```python
from build123d import *

# Parameters (mm, degrees)
BOSS_EXTRUDE1_DEPTH = 10
CHAMFER1_SIZE       = 1


with BuildPart() as part:
    # Sketch1 → Revolve1 (revolve)
    with BuildSketch(Plane.XY, mode=Mode.PRIVATE) as revolve1_sk:
        with BuildLine():
            Line((0, 0), (0, 15))
            Line((0, 15), (14.56869778, 15))
            ThreePointArc((14.56869778, 15), (15.493526394, 14.380384062), (15.27227791, 13.289384069))
            Line((15.27227791, 13.289384069), (12.24641987, 10.29348502))
            ThreePointArc((12.24641987, 10.29348502), (12.027075266, 9.967849524), (11.95, 9.582869089))
            Line((11.95, 9.582869089), (11.95, 5.417130911))
            ThreePointArc((11.95, 5.417130911), (12.027075266, 5.032150476), (12.24641987, 4.70651498))
            Line((12.24641987, 4.70651498), (15.27227791, 1.710615931))
            ThreePointArc((15.27227791, 1.710615931), (15.493526394, 0.619615938), (14.56869778, 0))
            Line((14.56869778, 0), (0, 0))
        make_face()
    revolve(revolve1_sk.sketch.rotate(Axis((-3.05, 12, 0), (0, -1, 0)), 180), axis=Axis((-3.05, 12, 0), (0, -1, 0)))

    # Sketch2 → Boss-Extrude1 (add)
    with BuildSketch(Plane(origin=(0, 15, 0), x_dir=(1, 0, 0), z_dir=(0, 1, 0))):
        with BuildLine():
            ThreePointArc((0, 0), (-0.18033103, 1.033198916), (-0.7, 1.94422221))
            Line((-0.7, 1.94422221), (-0.7, -1.94422221))
            ThreePointArc((-0.7, -1.94422221), (-0.18033103, -1.033198916), (0, 0))
        make_face()
    extrude(amount=-BOSS_EXTRUDE1_DEPTH)

    # Chamfer1
    chamfer1_edges = [part.edges().sort_by_distance(p)[0] for p in [
        (-4.083198916, 15, -2.86966897),
        (-0.7, 15, 0),
    ]]
    chamfer(chamfer1_edges, length=CHAMFER1_SIZE)


solid = part.part
```
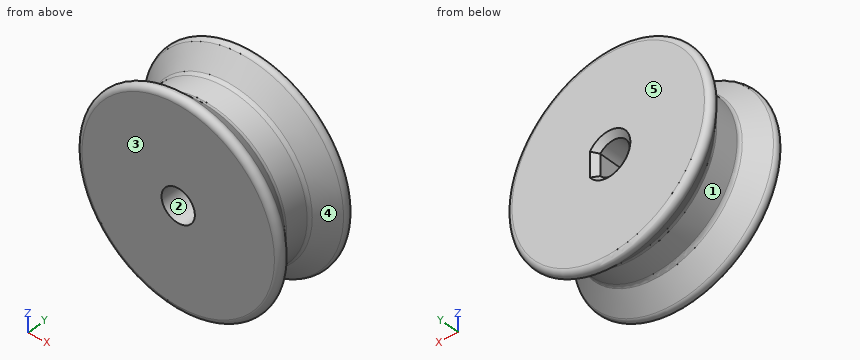
Source: CAD feature listing. Evaluate the final solid. Frame: model axes, mm. Face numbers are marked on the shaded views. A direction names the side the tool comes from. Coordinates: 2 decimals unless noted, no trailing zeros. Loops run counter-clockwise (first coordinate to the right, second up) from the corner with the lowest first, then second, coordinate; pieces in that order, holes last. Notation, with made-up numbers: (81, -38) -> (92, -38) arc R18 cw to (92, -33) -> close; hole circle Ø10 at (78, -23.5). An arc over 180 degrees is marked (long way). One line per item, written item: value. Start each with the question number.
Q1. Mould query, pull axis Y, two halves, no side actions, for the marked faces 1, 2 and 3. Classes: pulls with the +Y half, pulls with the -Y half, needs draft (parallel to the pull), parting line crosses it, or undercut.
Q2. Contact query for flat-ended pins moving along their axis: P1, Ø4, axis at y = 8, z = -10, coming from the -X side; P2, Ø2, axis at y = 2.5, z = 6.5, coming from the -X side; P3, Ø6, axis at y = 3, z = -6, coming from the +X side. Output: stop coordinate, or through.
Q3. Set-up query: the marked faces 4 and 5. Return all of +Z, -Z, +X, -X, +Y, -Y with unobstructed straight access to the full face (end or side cutting, diameter ignored); none if empty.
Q4. Line query: line 1 along Z through (x, y) = (-3.05, 6); line 2 along X through (y, z) = (1.5, -1.5); line 3 along Y through (x, z) = (4, -16.5). Output: solid intervals per line, ascending.
Q5. Section query B-B, the plane z = 0. Return the cut outline in (x, y), and give its area (3 significant figures).
Q6. Section query A-A, the plane x = -3.05. Return the cut outline in (y, z), and give its area (3 significant figures).
Q7. Section query C-C, the plane y = 1. Return the cut outline in (x, z), and give its area (3 significant figures).
Results:
1. face 1: undercut
1. face 2: needs draft
1. face 3: pulls with the -Y half
2. P1: x = -15.74
2. P2: x = -20.44
2. P3: x = 15.2
3. face 4: none
3. face 5: +Z, -Z, +X, -X, +Y
4. line 1: -15 to -3.05, 3.05 to 15
4. line 2: -21.47 to -5.71, -0.39 to 15.37
4. line 3: 0.05 to 2.09, 12.91 to 14.95
5. outline: (-21.37, 1.71) arc R1 ccw to (-20.67, 0) -> (-6.1, 0) -> (-6.1, 14) -> (-7.1, 15) -> (-20.67, 15) arc R1 ccw to (-21.37, 13.29) -> (-18.35, 10.29) arc R1 cw to (-18.05, 9.58) -> (-18.05, 5.42) arc R1 cw to (-18.35, 4.71) -> close; (-0.7, 5) -> (0, 5) -> (0, 0) -> (14.57, 0) arc R1 ccw to (15.27, 1.71) -> (12.25, 4.71) arc R1 cw to (11.95, 5.42) -> (11.95, 9.58) arc R1 cw to (12.25, 10.29) -> (15.27, 13.29) arc R1 ccw to (14.57, 15) -> (0.3, 15) -> (-0.7, 14) -> close
5. area: 410 mm^2
6. outline: (0, -17.62) arc R1 ccw to (1.71, -18.32) -> (4.71, -15.3) arc R1 cw to (5.42, -15) -> (9.58, -15) arc R1 cw to (10.29, -15.3) -> (13.29, -18.32) arc R1 ccw to (15, -17.62) -> (15, -4.05) -> (14, -3.05) -> (0, -3.05) -> close; (0, 3.05) -> (14, 3.05) -> (15, 4.05) -> (15, 17.62) arc R1 ccw to (13.29, 18.32) -> (10.29, 15.3) arc R1 cw to (9.58, 15) -> (5.42, 15) arc R1 cw to (4.71, 15.3) -> (1.71, 18.32) arc R1 ccw to (0, 17.62) -> close
6. area: 403 mm^2
7. outline: circle Ø37.24 at (-3.05, 0); hole circle Ø6.1 at (-3.05, 0)
7. area: 1,060 mm^2
